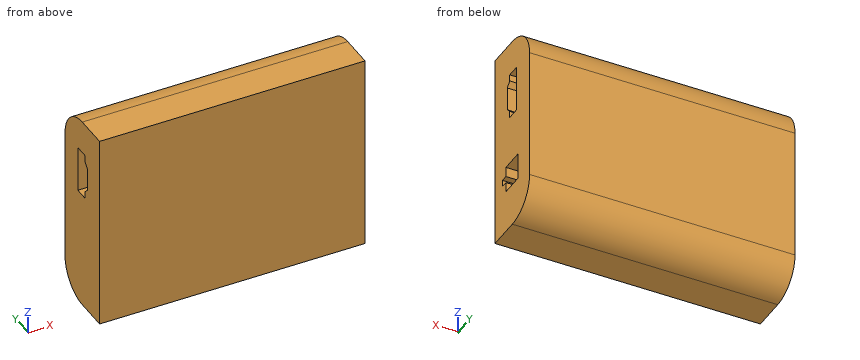
```python
from build123d import *

# Parameters (mm, degrees)
CROQUIS1_W              = 80
CROQUIS1_H              = 60
SALIENTE_EXTRUIR1_DEPTH = 20
CORTAR_EXTRUIR1_DEPTH   = 20
REDONDEO1_R             = 10
CORTAR_EXTRUIR2_DEPTH   = 20


with BuildPart() as part:
    # Croquis1 → Saliente-Extruir1 (new body)
    with BuildSketch(Plane(origin=(0, 0, 0), x_dir=(1, 0, 0), z_dir=(0, 1, 0))):
        with Locations((40, 30)):
            Rectangle(CROQUIS1_W, CROQUIS1_H)
    extrude(amount=SALIENTE_EXTRUIR1_DEPTH)

    # Croquis2 → Cortar-Extruir1 (cut)
    with BuildSketch(Plane(origin=(80, 0, 0), x_dir=(0, 0, -1), z_dir=(1, 0, 0))):
        Polygon((10, 12.52909884), (10, 8.52909884), (12, 8.52909884), (13.414213562, 7.114885277), (20.585786438, 7.114885277), (22, 8.52909884), (24, 8.52909884), (24, 12.52909884), align=None)
        Polygon((43.998137674, 6.318837227), (47, 6.318837227), (47, 13.165528149), (39, 13.165528149), (39, 6.318837227), (42.001862326, 6.318837227), (42.001862326, 4.318837227), (43.998137674, 4.318837227), align=None)
    extrude(amount=-CORTAR_EXTRUIR1_DEPTH, mode=Mode.SUBTRACT)

    # Redondeo1
    redondeo1_edges = [part.edges().sort_by_distance(p)[0] for p in [
        (40, 20, -60),
        (40, 20, 0),
    ]]
    fillet(redondeo1_edges, radius=REDONDEO1_R)

    # Croquis3 → Cortar-Extruir2 (cut)
    with BuildSketch(Plane.ZY):
        Polygon((-10, 12.52909884), (-24, 12.52909884), (-24, 8.52909884), (-22, 8.52909884), (-20.585786438, 7.114885277), (-13.414213562, 7.114885277), (-12, 8.52909884), (-10, 8.52909884), align=None)
    extrude(amount=-CORTAR_EXTRUIR2_DEPTH, mode=Mode.SUBTRACT)


solid = part.part
```
Check sheet for the modelled part. Datum: model origin and axes. Units: mm. Coordinates: 2 decimals unless noted, no trailing zeros. Loops run counter-clockwise (first coordinate to the right, second up) from the corner with the lowest first, then second, coordinate; pieces in that order, holes last. Notation, with made-up numbers: M 28,1.5 L 48,1.5 A8 ccw 48,7.5 Z; hole C 35,-31 d7. An arc over 180 degrees is marked long. Answer as a JSON object with one key per item and string values.
1. Sectioned sample at A-A on x = 75. Record the cut outline in (y, z).
Outcome:
{"outline": "M 0,-60 L 10,-60 A10 ccw 20,-50 L 20,-10 A10 ccw 10,0 L 0,0 Z; hole M 4.32,-44 L 6.32,-44 L 6.32,-47 L 13.17,-47 L 13.17,-39 L 6.32,-39 L 6.32,-42 L 4.32,-42 Z; hole M 7.11,-20.59 L 8.53,-22 L 8.53,-24 L 12.53,-24 L 12.53,-10 L 8.53,-10 L 8.53,-12 L 7.11,-13.41 Z"}
2. Sectioned sample at C-C on x = 14. Record the cut outline in (y, z).
Outcome:
{"outline": "M 0,-60 L 10,-60 A10 ccw 20,-50 L 20,-10 A10 ccw 10,0 L 0,0 Z; hole M 7.11,-20.59 L 8.53,-22 L 8.53,-24 L 12.53,-24 L 12.53,-10 L 8.53,-10 L 8.53,-12 L 7.11,-13.41 Z"}
3. Sectioned sample at D-D on y = 18. Record the cut outline in (x, z).
Outcome:
{"outline": "M 0,-56 L 80,-56 L 80,-4 L 0,-4 Z"}
4. Sectioned sample at B-B on z = -18. Record the cut outline in (x, y).
Outcome:
{"outline": "M 0,0 L 80,0 L 80,7.11 L 60,7.11 L 60,12.53 L 80,12.53 L 80,20 L 0,20 L 0,12.53 L 20,12.53 L 20,7.11 L 0,7.11 Z"}
5. Scan lines: L1, parallel to Z at x = 75.5, y = 5; L2, parallel to Z at x = 65, y = 8.25; L3, parallel to Z at x = 11, y = 9.25. Record each from-to range of solid material in increasing order. Write a range as from..to.
Outcome:
{"L1": "-60..-44, -42..0", "L2": "-60..-47, -39..-21.72, -12.28..0", "L3": "-60..-24, -10..0"}
